Read the model definition and answer for the solid it produces. Units are mm, in the model's axes. A direction names the side the tool comes from. Coordinates: 2 decimals unless noted, no trailing zeros. Loops run counter-clockwise (first coordinate to the right, second up) from the corner with the lowest first, then second, coordinate; pieces in that order, holes last. Notation, with made-up numbers: (44, 28) -> (58, 28) arc R12 cw to (58, 48) -> close; hole circle Ø6 at (0.25, -18.75). An arc over 180 degrees is marked (long way). Answer as a JSON object with one key per item and string values. Group by question number.
1) Section B-B, the plane x = 6 is taken. Give the vertices of the cut face in (y, z).
2) Section A-A, the plane y = 10 is taken. Give the vertices of the cut face in (x, z).
3) Determine the mould class of faces 3 (the face through (-7, 0, 3)), 4 (the face through (-23.97, 24.21, 1.48)), 5 (the face through (-27.859, -27.797, 1.521)) for opening direction X: released by +X, released by -X, zero draft, split by the parting line, or undercut.
4) Consider probe 1 along Y at (x, z) = (25, 2); probe 2 along X at (y, z) = (-6, 2.05); probe 3 along Y at (x, z) = (7, 1.1). Determine where each line is inside the solid, lowest interval first. Write a range as [from, to].
5) Which of the six approach directions +Z, -Z, +X, -X, +Y, -Y give full straight-line access (tool end or side, diameter ignored) to faces 1 (the face through (0, 29, 1)), 2 (the face through (17.5, 0, 2))?
6) Section C-C, the plane z = 1.8 is taken. Give the vertices of the cut face in (x, y), plus the area to 3 significant figures.
from build123d import *

# Parameters (mm, degrees)
ESBO_O1_W                    = 58
ESBO_O1_H                    = 58
RESSALTO_EXTRUS_O1_DEPTH     = 3
FURO_DE_DI_METRO_2_6_2_6_1_D = 2.6
PERFIL_CORTE_W               = 23
PERFIL_CORTE_H               = 12.4
CORTE_PRINCIPAL_DEPTH        = 85.236965894
FURO_DE_DI_METRO_3_0_3_1_D   = 3
FILETE1_R                    = 4


with BuildPart() as part:
    # Esboço1 → Ressalto-extrusão1 (new body)
    with BuildSketch(Plane.XY):
        Rectangle(ESBO_O1_W, ESBO_O1_H)
    extrude(amount=RESSALTO_EXTRUS_O1_DEPTH)

    # Furo de diâmetro Ø2.6 (2.6)1 (through all)
    with Locations(Plane.XY.offset(3)):
        with Locations((-25, 25), (25, 25), (25, -25), (-25, -25)):
            Hole(FURO_DE_DI_METRO_2_6_2_6_1_D / 2)

    # Perfil Corte → Corte Principal (cut, through all)
    with BuildSketch(Plane(origin=(-34.608741594, -26.143398661, 3), x_dir=(1, 0, 0), z_dir=(0, 0, 1))):
        with Locations((40.608741594, 26.143398661)):
            Rectangle(PERFIL_CORTE_W, PERFIL_CORTE_H)
    extrude(amount=-CORTE_PRINCIPAL_DEPTH, mode=Mode.SUBTRACT)

    # Furo de diâmetro Ø3.0 (3)1 (through all)
    with Locations(Plane(origin=(-55.097814602, -24.42830067, 3), x_dir=(1, 0, 0), z_dir=(0, 0, 1))):
        with Locations((61.097814602, 34.42830067), (61.097814602, 14.42830067)):
            Hole(FURO_DE_DI_METRO_3_0_3_1_D / 2)

    # Filete1
    filete1_edges = [part.edges().sort_by_distance(p)[0] for p in [
        (29, -29, 1.5),
        (-29, -29, 1.5),
        (-29, 29, 1.5),
        (29, 29, 1.5),
    ]]
    fillet(filete1_edges, radius=FILETE1_R)


solid = part.part
Determined:
{
 "1": {"outline": "(-29, 0) -> (-11.5, 0) -> (-11.5, 3) -> (-29, 3) -> close; (-8.5, 0) -> (-6.2, 0) -> (-6.2, 3) -> (-8.5, 3) -> close; (6.2, 0) -> (8.5, 0) -> (8.5, 3) -> (6.2, 3) -> close; (11.5, 0) -> (29, 0) -> (29, 3) -> (11.5, 3) -> close"},
 "2": {"outline": "(-29, 0) -> (4.5, 0) -> (4.5, 3) -> (-29, 3) -> close; (7.5, 0) -> (29, 0) -> (29, 3) -> (7.5, 3) -> close"},
 "3": {"face 3": "zero draft", "face 4": "undercut", "face 5": "released by -X"},
 "4": {"probe 1": "[-29, -26.3], [-23.7, 23.7], [26.3, 29]", "probe 2": "[-29, -5.5], [17.5, 29]", "probe 3": "[-29, -11.12], [-8.88, -6.2], [6.2, 8.88], [11.12, 29]"},
 "5": {"face 1": "+Z, -Z, +X, -X, +Y", "face 2": "+Z, -Z"},
 "6": {"outline": "(-29, -25) arc R4 ccw to (-25, -29) -> (25, -29) arc R4 ccw to (29, -25) -> (29, 25) arc R4 ccw to (25, 29) -> (-25, 29) arc R4 ccw to (-29, 25) -> close; hole circle Ø2.6 at (-25, -25); hole circle Ø2.6 at (-25, 25); hole (-5.5, -6.2) -> (17.5, -6.2) -> (17.5, 6.2) -> (-5.5, 6.2) -> close; hole circle Ø3 at (6, -10); hole circle Ø3 at (6, 10); hole circle Ø2.6 at (25, -25); hole circle Ø2.6 at (25, 25)", "area": "3,030 mm²"}
}
